from build123d import *

# Parameters (mm, degrees)
SKETCH1_W                     = 90
SKETCH1_H                     = 40
BASE_FLANGE1_DEPTH            = 0.5
EDGE_FLANGE1_STRIP_CUT_DEPTH  = 90
EDGE_FLANGE1_DEPTH            = 90
EDGE_FLANGE3_STRIP_CUT_DEPTH  = 90
EDGE_FLANGE3_DEPTH            = 90
EDGE_FLANGE2_STRIP_W          = 3
EDGE_FLANGE2_STRIP_H          = 0.5
EDGE_FLANGE2_STRIP_CUT_DEPTH  = 90
EDGE_FLANGE2_DEPTH            = 90
EDGE_FLANGE5_STRIP_W          = 3
EDGE_FLANGE5_STRIP_H          = 0.5
EDGE_FLANGE5_STRIP_CUT_DEPTH  = 90
EDGE_FLANGE5_DEPTH            = 90
EDGE_FLANGE7_DEPTH            = 48.292893219
EDGE_FLANGE8_DEPTH            = 48.292893219
CUT_EXTRUDE3_DEPTH            = 106.168160415
EDGE_FLANGE9_STRIP_W          = 3
EDGE_FLANGE9_STRIP_H          = 0.5
EDGE_FLANGE9_STRIP_CUT_DEPTH  = 28.3
EDGE_FLANGE9_DEPTH            = 28.3
EDGE_FLANGE10_STRIP_W         = 3
EDGE_FLANGE10_STRIP_H         = 0.5
EDGE_FLANGE10_STRIP_CUT_DEPTH = 28.2
EDGE_FLANGE10_DEPTH           = 28.2
SKETCH65_R                    = 1.5
CUT_EXTRUDE4_DEPTH            = 5


# Sheet-metal steps are written as plain solids
with BuildPart() as part:
    # Sketch1 → Base-Flange1 (new body)
    with BuildSketch(Plane(origin=(0, 0, 0), x_dir=(1, 0, 0), z_dir=(0, 1, 0))):
        Rectangle(SKETCH1_W, SKETCH1_H)
    extrude(amount=-BASE_FLANGE1_DEPTH)

    # Edge-Flange1 strip (across the edge) → Edge-Flange1 strip cut (cut)
    with BuildSketch(Plane(origin=(-45, 0, 20), x_dir=(0, -0.7071067811865513, -0.7071067811865438), z_dir=(1, 0, 0))):
        Polygon((-3.914213562, -4.621320344), (1.207106781, 0.5), (0.853553391, 0.853553391), (-4.267766953, -4.267766953), align=None)
    extrude(amount=EDGE_FLANGE1_STRIP_CUT_DEPTH, mode=Mode.SUBTRACT)

    # Edge-Flange1 section (across the edge) → Edge-Flange1 (add)
    with BuildSketch(Plane(origin=(-45, 0, 20), x_dir=(0, -0.7071067811865513, -0.7071067811865438), z_dir=(1, 0, 0))):
        with BuildLine():
            Line((-0.5, 1.207106781), (-0.5, 50))
            Line((-0.5, 50), (0, 50))
            Line((0, 50), (0, 1.207106781))
            ThreePointArc((0, 1.207106781), (0.308658284, 0.745167015), (0.853553391, 0.853553391))
            Line((0.853553391, 0.853553391), (1.207106781, 0.5))
            ThreePointArc((1.207106781, 0.5), (0.117316568, 0.283227249), (-0.5, 1.207106781))
        make_face()
    extrude(amount=EDGE_FLANGE1_DEPTH)

    # Edge-Flange3 strip (across the edge) → Edge-Flange3 strip cut (cut)
    with BuildSketch(Plane(origin=(45, 0, -20), x_dir=(0, 0.7071067811865562, 0.7071067811865388), z_dir=(-1, 0, 0))):
        Polygon((-2.328427125, 1.621320344), (-0.207106781, -0.5), (0.146446609, -0.146446609), (-1.974873734, 1.974873734), align=None)
    extrude(amount=EDGE_FLANGE3_STRIP_CUT_DEPTH, mode=Mode.SUBTRACT)

    # Edge-Flange3 section (across the edge) → Edge-Flange3 (add)
    with BuildSketch(Plane(origin=(45, 0, -20), x_dir=(0, 0.7071067811865562, 0.7071067811865388), z_dir=(-1, 0, 0))):
        with BuildLine():
            Line((-0.5, 0.207106781), (-0.5, 10))
            Line((-0.5, 10), (0, 10))
            Line((0, 10), (0, 0.207106781))
            ThreePointArc((0, 0.207106781), (0.038060234, 0.015765065), (0.146446609, -0.146446609))
            Line((0.146446609, -0.146446609), (-0.207106781, -0.5))
            ThreePointArc((-0.207106781, -0.5), (-0.423879533, -0.175576651), (-0.5, 0.207106781))
        make_face()
    extrude(amount=EDGE_FLANGE3_DEPTH)

    # Edge-Flange2 strip (across the edge) → Edge-Flange2 strip cut (cut)
    with BuildSketch(Plane(origin=(-45, 35.355339059, -15.355339059), x_dir=(0, -0.7071067811865511, 0.7071067811865439), z_dir=(1, 0, 0))):
        with Locations((-1, -0.25)):
            Rectangle(EDGE_FLANGE2_STRIP_W, EDGE_FLANGE2_STRIP_H)
    extrude(amount=EDGE_FLANGE2_STRIP_CUT_DEPTH, mode=Mode.SUBTRACT)

    # Edge-Flange2 section (across the edge) → Edge-Flange2 (add)
    with BuildSketch(Plane(origin=(-45, 35.355339059, -15.355339059), x_dir=(0, -0.7071067811865511, 0.7071067811865439), z_dir=(1, 0, 0))):
        with BuildLine():
            Line((-0.5, 0.5), (-0.5, 29))
            Line((-0.5, 29), (0, 29))
            Line((0, 29), (0, 0.5))
            ThreePointArc((0, 0.5), (0.146446609, 0.146446609), (0.5, 0))
            Line((0.5, 0), (0.5, -0.5))
            ThreePointArc((0.5, -0.5), (-0.207106781, -0.207106781), (-0.5, 0.5))
        make_face()
    extrude(amount=EDGE_FLANGE2_DEPTH)

    # Edge-Flange5 strip (across the edge) → Edge-Flange5 strip cut (cut)
    with BuildSketch(Plane(origin=(-45, 14.849242405, -35.861435714), x_dir=(0, 0.7071067811865416, 0.7071067811865535), z_dir=(1, 0, 0))):
        with Locations((-1, -0.25)):
            Rectangle(EDGE_FLANGE5_STRIP_W, EDGE_FLANGE5_STRIP_H)
    extrude(amount=EDGE_FLANGE5_STRIP_CUT_DEPTH, mode=Mode.SUBTRACT)

    # Edge-Flange5 section (across the edge) → Edge-Flange5 (add)
    with BuildSketch(Plane(origin=(-45, 14.849242405, -35.861435714), x_dir=(0, 0.7071067811865416, 0.7071067811865535), z_dir=(1, 0, 0))):
        with BuildLine():
            Line((-0.5, 0.5), (-0.5, 21))
            Line((-0.5, 21), (0, 21))
            Line((0, 21), (0, 0.5))
            ThreePointArc((0, 0.5), (0.146446609, 0.146446609), (0.5, 0))
            Line((0.5, 0), (0.5, -0.5))
            ThreePointArc((0.5, -0.5), (-0.207106781, -0.207106781), (-0.5, 0.5))
        make_face()
    extrude(amount=EDGE_FLANGE5_DEPTH)

    # Edge-Flange7 section (across the edge) → Edge-Flange7 (add)
    with BuildSketch(Plane(origin=(-45.5, 0.853553391, 19.146446609), x_dir=(1, 0, 0), z_dir=(0, 0.707106781186544, -0.7071067811865512))):
        with BuildLine():
            Line((-0.5, 0.5), (-0.5, 28.8))
            Line((-0.5, 28.8), (0, 28.8))
            Line((0, 28.8), (0, 0.5))
            ThreePointArc((0, 0.5), (0.146446609, 0.146446609), (0.5, 0))
            Line((0.5, 0), (0.5, -0.5))
            ThreePointArc((0.5, -0.5), (-0.207106781, -0.207106781), (-0.5, 0.5))
        make_face()
    extrude(amount=EDGE_FLANGE7_DEPTH)

    # Edge-Flange8 section (across the edge) → Edge-Flange8 (add)
    with BuildSketch(Plane(origin=(45.6, 35.001785669, -15.001785669), x_dir=(-1, 0, 0), z_dir=(0, -0.7071067811865439, 0.7071067811865512))):
        with BuildLine():
            Line((-0.5, 0.6), (-0.5, 28.8))
            Line((-0.5, 28.8), (0, 28.8))
            Line((0, 28.8), (0, 0.6))
            ThreePointArc((0, 0.6), (0.175735931, 0.175735931), (0.6, 0))
            Line((0.6, 0), (0.6, -0.5))
            ThreePointArc((0.6, -0.5), (-0.177817459, -0.177817459), (-0.5, 0.6))
        make_face()
    extrude(amount=EDGE_FLANGE8_DEPTH)

    # Sketch52 → Cut-Extrude3 (cut, through all)
    with BuildSketch(Plane.ZY.offset(46)):
        Polygon((-20.229350596, -0.5), (17.792893219, -0.5), (-1.218228689, -19.511121908), align=None)
    extrude(amount=-CUT_EXTRUDE3_DEPTH, mode=Mode.SUBTRACT)

    # Edge-Flange9 strip (across the edge) → Edge-Flange9 strip cut (cut)
    with BuildSketch(Plane(origin=(-45.5, 14.637110371, -35.366460967), x_dir=(3.347797797820495e-15, -0.7071067811865438, 0.7071067811865515), z_dir=(0, 0.7071067811865515, 0.7071067811865438))):
        with Locations((-0.5, -0.25)):
            Rectangle(EDGE_FLANGE9_STRIP_W, EDGE_FLANGE9_STRIP_H)
    extrude(amount=EDGE_FLANGE9_STRIP_CUT_DEPTH, mode=Mode.SUBTRACT)

    # Edge-Flange9 section (across the edge) → Edge-Flange9 (add)
    with BuildSketch(Plane(origin=(-45.5, 14.637110371, -35.366460967), x_dir=(3.347797797820495e-15, -0.7071067811865438, 0.7071067811865515), z_dir=(0, 0.7071067811865515, 0.7071067811865438))):
        with BuildLine():
            Line((0, 0.5), (0, 10))
            Line((0, 10), (0.5, 10))
            Line((0.5, 10), (0.5, 0.5))
            ThreePointArc((0.5, 0.5), (0.646446609, 0.146446609), (1, 0))
            Line((1, 0), (1, -0.5))
            ThreePointArc((1, -0.5), (0.292893219, -0.207106781), (0, 0.5))
        make_face()
    extrude(amount=EDGE_FLANGE9_DEPTH)

    # Edge-Flange10 strip (across the edge) → Edge-Flange10 strip cut (cut)
    with BuildSketch(Plane(origin=(45.6, 34.5775216, -15.426049737), x_dir=(-3.491481338843137e-15, -0.7071067811865434, 0.7071067811865518), z_dir=(3.4448409452021724e-15, -0.7071067811865518, -0.7071067811865434))):
        with Locations((-0.5, -0.25)):
            Rectangle(EDGE_FLANGE10_STRIP_W, EDGE_FLANGE10_STRIP_H)
    extrude(amount=EDGE_FLANGE10_STRIP_CUT_DEPTH, mode=Mode.SUBTRACT)

    # Edge-Flange10 section (across the edge) → Edge-Flange10 (add)
    with BuildSketch(Plane(origin=(45.6, 34.5775216, -15.426049737), x_dir=(-3.491481338843137e-15, -0.7071067811865434, 0.7071067811865518), z_dir=(3.4448409452021724e-15, -0.7071067811865518, -0.7071067811865434))):
        with BuildLine():
            Line((0, 0.5), (0, 10))
            Line((0, 10), (0.5, 10))
            Line((0.5, 10), (0.5, 0.5))
            ThreePointArc((0.5, 0.5), (0.646446609, 0.146446609), (1, 0))
            Line((1, 0), (1, -0.5))
            ThreePointArc((1, -0.5), (0.292893219, -0.207106781), (0, 0.5))
        make_face()
    extrude(amount=EDGE_FLANGE10_DEPTH)

    # Sketch65 → Cut-Extrude4 (cut)
    with BuildSketch(Plane.XZ.offset(0.5)):
        with Locations(Location((-41, 9.591937881, 0), (0, 0, 270))):
            Circle(SKETCH65_R)
        with Locations(Location((41, 9.591937881, 0), (0, 0, 90))):
            Circle(SKETCH65_R)
        with Locations(Location((-41, -12.92766953, 0), (0, 0, 270))):
            Circle(SKETCH65_R)
        with Locations(Location((41, -12.92766953, 0), (0, 0, 90))):
            Circle(SKETCH65_R)
    extrude(amount=-CUT_EXTRUDE4_DEPTH, mode=Mode.SUBTRACT)


solid = part.part
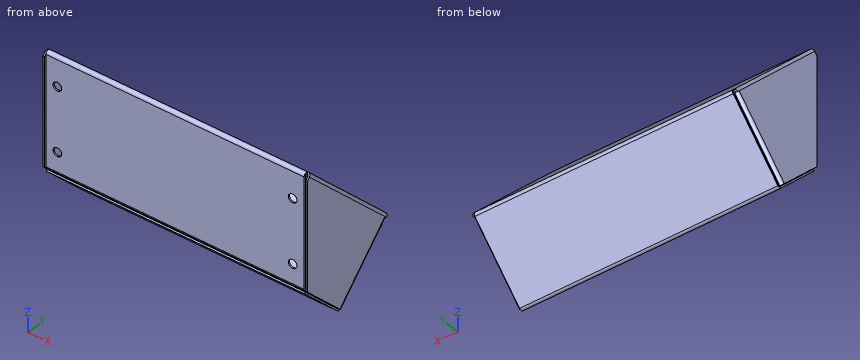
Can you work these out from the model? Positions are in its coordinate system, mm. Round coordinates to 2 decimals unless told otherwise and drop trailing zeros. Write each loop counter-clockwise with the first axis right and the second up, starting at its lowest first coordinate (ties: lowest second). Pieces come first, ordered by that corner, then holes. Notation, with made-up numbers: (-32.5, 55) -> (5.5, 55) arc R27 cw to (5.5, 91) -> close; hole circle Ø4 at (89, 1.5). An arc over 180 degrees is marked (long way). One line per question, with ' | ' between items. Start each with the question number.
1) Suppose I cut it at B-B on x = 14. Write out the boundary of the cut face in (y, z).
2) I need wall thicknesses on line 1 (X direction, y = 9, z = -23); line 2 (Y direction, x = 24.5, z = -27); line 3 (Y direction, x = -37.5, z = -25). Which ranges of each line are inside material? Lowest first, please. Write a range as [from, to].
3) I'm going to push flat-ended pins straight in: P1, Ø2.5, axis at x = -41, z = -12.93, coming from the -Y side; P2, Ø2, axis at x = 15, y = 6, coming from the +Z side; P3, Ø1.8, axis at x = 41, z = 9.59, coming from the -Y side. Where does each tip first touch, or does it pass through?
4) Suppose I cut it at A-A on x = 41. Count the separate pieces of the cut face and the enclosed holes in it, then the cut area to 3 significant figures.
Return value:
1) outline: (-0.5, -19.79) arc R1 ccw to (-0.21, -20.5) -> (6.72, -27.42) -> (7.07, -27.07) -> (0.15, -20.15) arc R0.5 cw to (0, -19.79) -> (0, 18.79) arc R0.5 cw to (0.85, 19.15) -> (35, -15) arc R0.5 cw to (35, -15.71) -> (15.2, -35.51) arc R0.5 cw to (14.5, -35.51) -> (0, -21.01) -> (-0.35, -21.37) -> (14.14, -35.86) arc R1 ccw to (15.56, -35.86) -> (35.36, -16.06) arc R1 ccw to (35.36, -14.65) -> (1.21, 19.5) arc R1 ccw to (-0.5, 18.79) -> close
2) line 1: x = [-46, -45.5], [45.6, 46.1] | line 2: y = [5.28, 5.99], [6.29, 7], [23.71, 24.42] | line 3: y = [3.28, 3.99], [4.29, 5], [24.3, 25], [25.71, 26.42]
3) P1: stops at y = 31.68 | P2: stops at z = 15.71 | P3: stops at y = 9.51
4) separate pieces: 4 | enclosed holes: 0 | area: 86.0 mm2
